Design review of the part shown in the three views and the two pictorial views. Dimensions are in mm from the part's minimum x, y and z. A direction names the side the tool comes from. Coordinates: 2 decimals unless noted, no trailing zeros. Order: outer loops, then holes, each group sorted by start corner. A loop starts at its lowest first (then second) coordinate and runs counter-clockwise, first axis right, second up. Notation, with made-up numbers: M 6.5,56 L 29.5,56 A7 ccw 29.5,69 Z; hole C 76,42.5 d6. An arc over 180 degrees is marked long. Use CSV: the item, a comma, the result in double quotes.
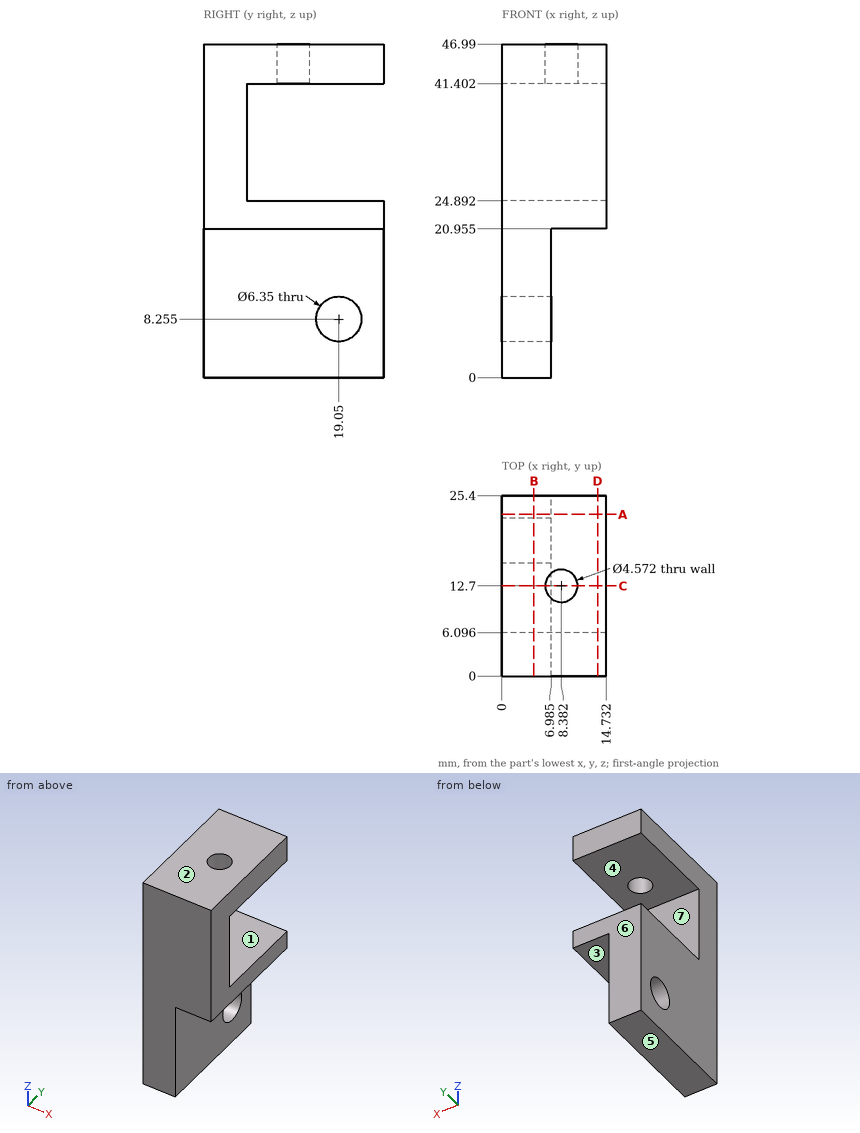
(1) The part is to be moulded in two halves that separate along Z. For the marked faces 4, 5, 6 and 7, say which applies: pulls with the +Z half, pulls with the -Z half, needs draft (parallel to the pull), parting line crosses it, or undercut.
The answers:
face 4,"undercut"
face 5,"pulls with the -Z half"
face 6,"needs draft"
face 7,"undercut"
(2) For the marked faces 1, 2 and 3, list the 3-axis set-ups (+Z, -Z, +X, -X, +Y, -Y) from which the entire face can be reached by the end or side of a thin tool; tool diameter is ignored.
The answers:
face 1,"+X, -X, +Y"
face 2,"+Z, +X, -X, +Y, -Y"
face 3,"-Z, +X, +Y, -Y"
(3) Add section D-D on x = 13.5. State the section outline as (y, z) points (3 decimals).
The answers:
outline,"M 0,20.955 L 25.4,20.955 L 25.4,24.892 L 6.096,24.892 L 6.096,41.402 L 25.4,41.402 L 25.4,46.99 L 0,46.99 Z"
(4) Add section B-B on x = 4.5. State the section outline as (y, z) points (3 decimals), and give its area (3 significant figures).
The answers:
outline,"M 0,0 L 25.4,0 L 25.4,24.892 L 6.096,24.892 L 6.096,41.402 L 25.4,41.402 L 25.4,46.99 L 0,46.99 Z; hole C 19.05,8.255 d6.35"
area,"843 mm2"
(5) Add section C-C on y = 12.7. State the section outline as (x, z) points (3 decimals).
The answers:
outline,"M 0,0 L 6.985,0 L 6.985,20.955 L 14.732,20.955 L 14.732,24.892 L 0,24.892 Z; M 0,41.402 L 6.096,41.402 L 6.096,46.99 L 0,46.99 Z; M 10.668,41.402 L 14.732,41.402 L 14.732,46.99 L 10.668,46.99 Z"
(6) Clearance check with flat-ended pins moving along their axes: P1, Ø3, axis at x = 9, z = 32.5, coming from the +Y side; P2, Ø6, axis at x = 11, y = 9, coming from the -Z side (3 decimals). State where each tip first meets the part, or that it passes through.
The answers:
P1,"stops at y = 6.1"
P2,"stops at z = 20.955"
(7) Add section A-A on y = 22.75. State the section outline as (x, z) points (3 decimals).
The answers:
outline,"M 0,0 L 6.985,0 L 6.985,20.955 L 14.732,20.955 L 14.732,24.892 L 0,24.892 Z; M 0,41.402 L 14.732,41.402 L 14.732,46.99 L 0,46.99 Z"
(8) Wall thickness on probe 1 along Z at (x, y) = (12.75, 21.25) (3 decimals); probe 2 along Z at (x, y) = (1.75, 16.75); probe 3 along Z at (x, y) = (6.75, 20.75): over which ranges is each line inside the solid? List them lowest first.
The answers:
probe 1,"z = 20.955 to 24.892, 41.402 to 46.99"
probe 2,"z = 0 to 6.07, 10.44 to 24.89, 41.4 to 46.99"
probe 3,"z = 0 to 5.57, 10.94 to 24.89, 41.4 to 46.99"
